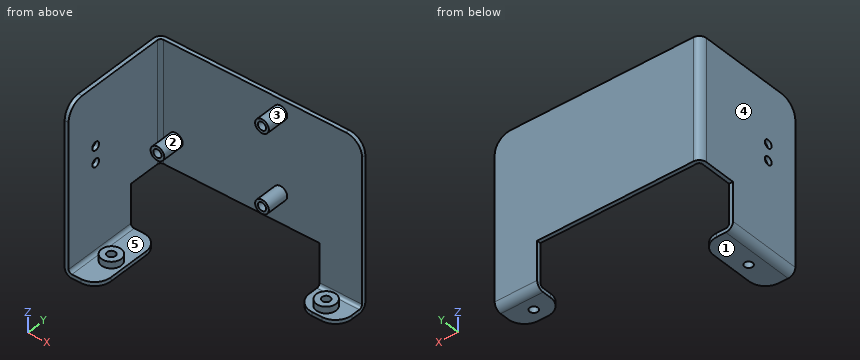
from build123d import *

# Parameters (mm, degrees)
SM_BASE_FLANGE_1_DEPTH           = 1.2
SKETCH_9_R                       = 2.1
EXTRUDE_1_DEPTH                  = 6.8
HOLE_WIZARD_M3_1_D               = 2.5
HOLE_WIZARD_M3_1_DEPTH           = 3
SM_EDGE_FLANGE_1_STRIP_W         = 6.8
SM_EDGE_FLANGE_1_STRIP_H         = 1.2
SM_EDGE_FLANGE_1_STRIP_CUT_DEPTH = 13
SM_EDGE_FLANGE_1_DEPTH           = 13
SM_EDGE_FLANGE_1_FLAT_DEPTH      = 1.2
SKETCH_15_R                      = 3
EXTRUDE_2_DEPTH                  = 2
HOLE_WIZARD_M3_2_D               = 2.5
SM_EDGE_FLANGE_4_STRIP_W         = 6.8
SM_EDGE_FLANGE_4_STRIP_H         = 1.2
SM_EDGE_FLANGE_4_STRIP_CUT_DEPTH = 37
SM_EDGE_FLANGE_4_DEPTH           = 37
SM_EDGE_FLANGE_4_FLAT_DEPTH      = 1.2
SM_EDGE_FLANGE_5_STRIP_W         = 6.8
SM_EDGE_FLANGE_5_STRIP_H         = 1.2
SM_EDGE_FLANGE_5_STRIP_CUT_DEPTH = 23
SM_EDGE_FLANGE_5_DEPTH           = 23
SM_EDGE_FLANGE_5_FLAT_DEPTH      = 1.2
SKETCH_26_R                      = 3
EXTRUDE_3_DEPTH                  = 2
HOLE_WIZARD_M3_3_D               = 2.5
CUT_EXTRUDE_1_REACH              = 78.751
SKETCH_29_R                      = 1.25


# Sheet-metal steps are written as plain solids
with BuildPart() as part:
    # Sketch 1 → 基体-法兰1 (new body)
    with BuildSketch(Plane(origin=(0, 0, 0), x_dir=(1, 0, 0), z_dir=(0, 1, 0))):
        with BuildLine():
            Line((18.5, 24.605976874), (31.5, 24.605976874))
            Line((31.5, 24.605976874), (31.5, -21.394023126))
            ThreePointArc((31.5, -21.394023126), (30.035533906, -24.929557032), (26.5, -26.394023126))
            Line((26.5, -26.394023126), (-31.5, -26.394023126))
            Line((-31.5, -26.394023126), (-31.5, 10.605976874))
            Line((-31.5, 10.605976874), (18.5, 10.605976874))
            Line((18.5, 10.605976874), (18.5, 24.605976874))
        make_face()
    extrude(amount=-SM_BASE_FLANGE_1_DEPTH)

    # 草图9 → 凸台-拉伸1 (add)
    with BuildSketch(Plane.XZ.offset(1.2)):
        with Locations(Location((-25.5, -1.605976874, 0), (0, 0, 270))):
            Circle(SKETCH_9_R)
        with Locations(Location((6.5, 22.394023126, 0), (0, 0, 270))):
            Circle(SKETCH_9_R)
        with Locations(Location((6.5, -1.605976874, 0), (0, 0, 270))):
            Circle(SKETCH_9_R)
    extrude(amount=EXTRUDE_1_DEPTH)

    # M3 螺纹孔1
    with Locations(Plane(origin=(0, -8, 0), x_dir=(-1, 0, 0), z_dir=(0, -1, 0))):
        with Locations((-6.5, 1.605976874), (25.5, 1.605976874), (-6.5, -22.394023126)):
            Hole(HOLE_WIZARD_M3_1_D / 2, depth=HOLE_WIZARD_M3_1_DEPTH)

    # 边线-法兰1 strip (across the edge) → 边线-法兰1 strip cut (cut)
    with BuildSketch(Plane(origin=(18.5, -1.2, -24.605976874), x_dir=(0, 0, 1), z_dir=(1, 0, 0))):
        with Locations((-1.2, -0.6)):
            Rectangle(SM_EDGE_FLANGE_1_STRIP_W, SM_EDGE_FLANGE_1_STRIP_H)
    extrude(amount=SM_EDGE_FLANGE_1_STRIP_CUT_DEPTH, mode=Mode.SUBTRACT)

    # 边线-法兰1 bend section (across the edge) → 边线-法兰1 (add)
    with BuildSketch(Plane(origin=(18.5, -1.2, -24.605976874), x_dir=(0, 0, 1), z_dir=(1, 0, 0))):
        with BuildLine():
            Line((0, 1), (1.2, 1))
            ThreePointArc((1.2, 1), (1.492893219, 0.292893219), (2.2, 0))
            Line((2.2, 0), (2.2, -1.2))
            ThreePointArc((2.2, -1.2), (0.644365081, -0.555634919), (0, 1))
        make_face()
    extrude(amount=SM_EDGE_FLANGE_1_DEPTH)

    # 边线-法兰1 profile (on flange) → 边线-法兰1 flat (add)
    with BuildSketch(Plane(origin=(0, -1.2, -24.605976874), x_dir=(1, 0, 0), z_dir=(0, 0, -1))):
        with BuildLine():
            Line((31.5, 1), (31.5, 3.8))
            ThreePointArc((31.5, 3.8), (30.035533906, 7.335533906), (26.5, 8.8))
            Line((26.5, 8.8), (23.5, 8.8))
            ThreePointArc((23.5, 8.8), (19.964466094, 7.335533906), (18.5, 3.8))
            Line((18.5, 3.8), (18.5, 1))
            Line((18.5, 1), (31.5, 1))
        make_face()
    extrude(amount=-SM_EDGE_FLANGE_1_FLAT_DEPTH)

    # 草图15 → 凸台-拉伸2 (add)
    with BuildSketch(Plane.XY.offset(-23.405976874)):
        with Locations((24.5, -6)):
            Circle(SKETCH_15_R)
    extrude(amount=EXTRUDE_2_DEPTH)

    # M3 螺纹孔2 (through all)
    with Locations(Plane.XY.offset(-21.405976874)):
        with Locations((24.5, -6)):
            Hole(HOLE_WIZARD_M3_2_D / 2)

    # 边线-法兰4 strip (across the edge) → 边线-法兰4 strip cut (cut)
    with BuildSketch(Plane(origin=(-31.5, -1.2, 26.394023126), x_dir=(1, 0, 0), z_dir=(0, 0, -1))):
        with Locations((-1.2, -0.6)):
            Rectangle(SM_EDGE_FLANGE_4_STRIP_W, SM_EDGE_FLANGE_4_STRIP_H)
    extrude(amount=SM_EDGE_FLANGE_4_STRIP_CUT_DEPTH, mode=Mode.SUBTRACT)

    # 边线-法兰4 bend section (across the edge) → 边线-法兰4 (add)
    with BuildSketch(Plane(origin=(-31.5, -1.2, 26.394023126), x_dir=(1, 0, 0), z_dir=(0, 0, -1))):
        with BuildLine():
            Line((0, 1), (1.2, 1))
            ThreePointArc((1.2, 1), (1.492893219, 0.292893219), (2.2, 0))
            Line((2.2, 0), (2.2, -1.2))
            ThreePointArc((2.2, -1.2), (0.644365081, -0.555634919), (0, 1))
        make_face()
    extrude(amount=SM_EDGE_FLANGE_4_DEPTH)

    # 边线-法兰4 profile (on flange) → 边线-法兰4 flat (add)
    with BuildSketch(Plane(origin=(-31.5, -1.2, 0), x_dir=(0, 0, -1), z_dir=(-1, 0, 0))):
        with BuildLine():
            Line((-26.394023126, 1), (10.605976874, 1))
            Line((10.605976874, 1), (10.605976874, 10.8))
            Line((10.605976874, 10.8), (24.605976874, 10.8))
            Line((24.605976874, 10.8), (24.605976874, 33.8))
            Line((24.605976874, 33.8), (-21.394023126, 33.8))
            ThreePointArc((-21.394023126, 33.8), (-24.929557032, 32.335533906), (-26.394023126, 28.8))
            Line((-26.394023126, 28.8), (-26.394023126, 1))
        make_face()
    extrude(amount=-SM_EDGE_FLANGE_4_FLAT_DEPTH)

    # 边线-法兰5 strip (across the edge) → 边线-法兰5 strip cut (cut)
    with BuildSketch(Plane(origin=(-30.3, -35, -24.605976874), x_dir=(0, 0, 1), z_dir=(0, 1, 0))):
        with Locations((-1.2, -0.6)):
            Rectangle(SM_EDGE_FLANGE_5_STRIP_W, SM_EDGE_FLANGE_5_STRIP_H)
    extrude(amount=SM_EDGE_FLANGE_5_STRIP_CUT_DEPTH, mode=Mode.SUBTRACT)

    # 边线-法兰5 bend section (across the edge) → 边线-法兰5 (add)
    with BuildSketch(Plane(origin=(-30.3, -35, -24.605976874), x_dir=(0, 0, 1), z_dir=(0, 1, 0))):
        with BuildLine():
            Line((0, 1), (1.2, 1))
            ThreePointArc((1.2, 1), (1.492893219, 0.292893219), (2.2, 0))
            Line((2.2, 0), (2.2, -1.2))
            ThreePointArc((2.2, -1.2), (0.644365081, -0.555634919), (0, 1))
        make_face()
    extrude(amount=SM_EDGE_FLANGE_5_DEPTH)

    # 边线-法兰5 profile (on flange) → 边线-法兰5 flat (add)
    with BuildSketch(Plane(origin=(-30.3, 0, -24.605976874), x_dir=(0, 1, 0), z_dir=(0, 0, -1))):
        with BuildLine():
            ThreePointArc((-12, 3.8), (-13.464466094, 7.335533906), (-17, 8.8))
            Line((-17, 8.8), (-30, 8.8))
            ThreePointArc((-30, 8.8), (-33.535533906, 7.335533906), (-35, 3.8))
            Line((-35, 3.8), (-35, 1))
            Line((-35, 1), (-12, 1))
            Line((-12, 1), (-12, 3.8))
        make_face()
    extrude(amount=-SM_EDGE_FLANGE_5_FLAT_DEPTH)

    # 草图26 → 凸台-拉伸3 (add)
    with BuildSketch(Plane.XY.offset(-23.405976874)):
        with Locations(Location((-25.5, -25, 0), (0, 0, 180))):
            Circle(SKETCH_26_R)
    extrude(amount=EXTRUDE_3_DEPTH)

    # M3 螺纹孔3 (through all)
    with Locations(Plane.XY.offset(-21.405976874)):
        with Locations((-25.5, -25)):
            Hole(HOLE_WIZARD_M3_3_D / 2)

    # 草图29 → 切除-拉伸1 (cut, up to next)
    with BuildSketch(Plane.ZY.offset(31.5), mode=Mode.PRIVATE) as cut_extrude_1_sk1:
        with Locations(Location((3.394023126, -25, 0), (0, 0, 270))):
            Circle(SKETCH_29_R)
    cut_extrude_1_tool1 = extrude(cut_extrude_1_sk1.sketch, amount=-CUT_EXTRUDE_1_REACH, mode=Mode.PRIVATE) & part.part
    # 草图29 → 切除-拉伸1 (cut, up to next)
    with BuildSketch(Plane.ZY.offset(31.5), mode=Mode.PRIVATE) as cut_extrude_1_sk2:
        with Locations(Location((8.394023126, -25, 0), (0, 0, 270))):
            Circle(SKETCH_29_R)
    cut_extrude_1_tool2 = extrude(cut_extrude_1_sk2.sketch, amount=-CUT_EXTRUDE_1_REACH, mode=Mode.PRIVATE) & part.part
    add(cut_extrude_1_tool1.solids().sort_by_distance((-31.5, -25, 3.394023))[0], mode=Mode.SUBTRACT)
    add(cut_extrude_1_tool2.solids().sort_by_distance((-31.5, -25, 8.394023))[0], mode=Mode.SUBTRACT)


solid = part.part
Can you work these out from the model? Positions are in its coordinate system, mm. Face numbers are marked on the shaded views. A direction names the side the tool comes from. Round coordinates to 2 decimals unless told otherwise and drop trailing zeros. Write each loop counter-clockwise with the first axis right and the second up, starting at its lowest first coordinate (ties: lowest second). Pieces come first, ordered by that corner, then holes. Notation, with made-up numbers: (-39, -11.5) - (18, -11.5) arc R24 ccw to (18, 19.5) - close; hole circle Ø8 at (14.25, 84). An arc over 180 degrees is marked (long way). Write each question's results on one line, items separated by ' | '. Start each with the question number.
1) Please list where these lines run through material, in increasing order: line 1 (Y direction, x = -23.5, z = 2); line 2 (X direction, y = -30, z = -16.5); line 3 (Z direction, x = -26, y = -6.5).
2) Which directions (+Z, -Z, +X, -X, +Y, -Y) give clear straight access to the entire face, cutting with the end or side of a thin tool? Please do the marked faces 1 and 2.
3) For pin 1 Ø4 at (x, z) = (-25.5, -1.61) entering from -Y; pin 2 Ø1.5 at (x, z) = (6.5, -1.61) entering from +Y; pin 3 Ø1 at (y, z) = (-25.5, -24) entering from +X; pin 4 Ø2.5 at (x, y) = (-25, -19) entering from +Z, each with a flat end and sliding along its axis, tell me the tip position at first contact or that it passes through.
4) Suppose I cut it at D-D (z = 17). List the corners of the cut face in (x, y) for me.
5) Suppose I cut it at A-A (x = 24.5). List the corners of the cut face in (y, z) for me, and give its area (3 significant figures).
6) We'd pull the mould along Z, two halves only. Please class the marked faces 3, 4 and 5: released by +Z, released by -Z, zero draft, split by the parting line, or undercut.
7) Suppose I cut it at C-C (y = -25). List the corners of the cut face in (x, z) for me.
8) Suppose I cut it at B-B (y = -6). Give the number of separate pieces and of enclosed holes in the cut face, and give its area (3 significant figures).
Here are the results:
1) line 1: y = -1.2 to 0 | line 2: x = -31.5 to -30.3 | line 3: z = -3.65 to -2.75, -0.46 to 0.43
2) face 1: -Z, +X, -X, +Y, -Y | face 2: -Y
3) pin 1: stops at y = -8 | pin 2: stops at y = 0 | pin 3: stops at x = -21.5 | pin 4: stops at z = -23.41
4) outline: (-31.5, -35) - (-30.3, -35) - (-30.3, -2.2) arc R1 cw to (-29.3, -1.2) - (31.5, -1.2) - (31.5, 0) - (-29.3, 0) arc R2.2 ccw to (-31.5, -2.2) - close
5) outline: (-10, -24.61) - (-7.25, -24.61) - (-7.25, -21.41) - (-9, -21.41) - (-9, -23.41) - (-10, -23.41) - close; (-4.75, -24.61) - (-2.2, -24.61) arc R2.2 ccw to (0, -22.41) - (0, 26.39) - (-1.2, 26.39) - (-1.2, -22.41) arc R1 cw to (-2.2, -23.41) - (-3, -23.41) - (-3, -21.41) - (-4.75, -21.41) - close | area: 74.9 mm2
6) face 3: undercut | face 4: zero draft | face 5: released by +Z
7) outline: (-31.5, -22.41) arc R2.2 ccw to (-29.3, -24.61) - (-26.75, -24.61) - (-26.75, -21.41) - (-28.5, -21.41) - (-28.5, -23.41) - (-29.3, -23.41) arc R1 cw to (-30.3, -22.41) - (-30.3, 2.14) - (-31.5, 2.14) - close; (-31.5, 4.64) - (-30.3, 4.64) - (-30.3, 7.14) - (-31.5, 7.14) - close; (-31.5, 9.64) - (-30.3, 9.64) - (-30.3, 26.39) - (-31.5, 26.39) - close; (-24.25, -24.61) - (-21.5, -24.61) - (-21.5, -23.41) - (-22.5, -23.41) - (-22.5, -21.41) - (-24.25, -21.41) - close
8) separate pieces: 6 | enclosed holes: 3 | area: 90.6 mm2
